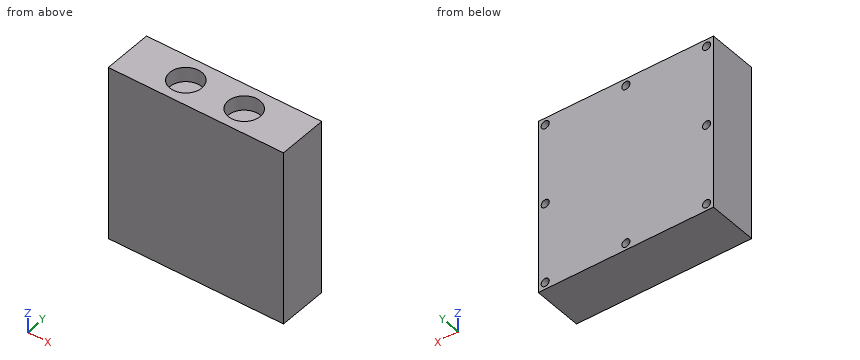
Autodesk Inventor part; units mm, degrees
ref_plane "YZ Plane" through (0, 0, 0) normal (1, 0, 0) x (0, 1, 0)
ref_plane "XZ Plane" through (0, 0, 0) normal (0, 1, 0) x (-1, 0, 0)
ref_plane "XY Plane" through (0, 0, 0) normal (0, 0, 1) x (1, 0, 0)
sketch "Sketch1" plane through (0, 0, 0) normal (0, 1, 0) x (-1, 0, 0)
  line L0 (0, 0) -> (-76.2, 0)
  line L1 (-76.2, 0) -> (-76.2, -76.2)
  line L2 (-76.2, -76.2) -> (0, -76.2)
  line L3 (0, -76.2) -> (0, 0)
  dimension "d0" = 76.2
  dimension "d1" = 76.2
extrude "Extrusion1" add sketch "Sketch1" along normal blind 21.59
sketch "Sketch2" plane through (0, 21.59, 0) normal (0, 1, 0) x (1, 0, 0)
  line L0 (76.2, 76.2) -> (0, 76.2)
  line L1 (38.1, 76.2) -> (38.1, 73.1774)
  line L2 (0, 76.2) -> (0, 0)
  line L3 (0, 38.1) -> (3.0226, 38.1)
  line L4 (0, 0) -> (76.2, 0)
  line L5 (38.1, 0) -> (38.1, 3.0226)
  line L6 (76.2, 0) -> (76.2, 76.2)
  line L7 (76.2, 38.1) -> (73.1774, 38.1)
  circle A0 centre (3.0226, 73.1774) radius 1.7526
  circle A1 centre (73.1774, 3.0226) radius 1.7526
  circle A2 centre (73.1774, 73.1774) radius 1.7526
  circle A3 centre (38.1, 3.0226) radius 1.7526
  circle A4 centre (3.0226, 38.1) radius 1.7526
  circle A5 centre (38.1, 73.1774) radius 1.7526
  circle A6 centre (3.0226, 3.0226) radius 1.7526
  circle A7 centre (73.1774, 38.1) radius 1.7526
  dimension "d5" = 3.0226
  dimension "d6" = 3.0226
  dimension "d7" = 3.0226
  dimension "d8" = 3.0226
  dimension "d9" = 3.5052
  dimension "d10" = 3.5052
  dimension "d11" = 3.5052
  dimension "d12" = 3.5052
  dimension "d13" = 3.5052
  dimension "d14" = 3.5052
  dimension "d15" = 3.5052
  dimension "d16" = 3.5052
extrude "Extrusion2" cut sketch "Sketch2" against normal blind 11.43 contours A5 | A4 | A3 | A7 | A0 | A1 | A2 | A6
sketch "Sketch3" plane through (0, 0, 0) normal (0, 0, 1) x (1, 0, 0)
  line L0 (0, 0) -> (0, 21.59)
  circle A0 centre (25.4, 10.795) radius 6.985
  circle A1 centre (50.8, 10.795) radius 6.985
  dimension "d21" = 13.97
  dimension "d22" = 13.97
extrude "Extrusion3" cut sketch "Sketch3" against normal blind 6.35
properties part number "water_block_top"
Geometry check sheet. Reference: the model listing, model coordinates, mm. Round coordinates to 2 decimals unless told otherwise and drop trailing zeros. Order: outer loops, then holes, each group sorted by start corner. A loop starts at its lowest first (then second) coordinate and runs counter-clockwise, first axis right, second up. Notation, with made-up numbers: (87.5, 39.5) -> (111.5, 39.5) arc R11 cw to (111.5, 55.5) -> close; hole circle Ø2 at (-10.5, 76). An arc over 180 degrees is marked (long way). Return JSON: item names as keys, results as strings. Group by question number.
Q1. Section check B-B, the plane z = -38.1. Record the boundary of the cut face in (x, y), plus the area to 3 significant figures.
Q2. Section check C-C, the plane x = 50.8. Record the boundary of the cut face in (y, z), plus the area to 3 significant figures.
Q3. Gauge pin test, flat ends, axial feed: pin 1 (2 mm diameter, centred on x = 3.02, z = -73.18, fed in from -Y); pin 2 (7 mm diameter, centred on x = 52.5, y = 12.5, fed in from +Z); pin 3 (1.8 mm diameter, centred on x = 2.5, z = -38, fed in from +Y). Record the tip position at first contact, or that the pin passes through.
Q4. Material ranges on probe 1 along X at (y, z) = (18.75, -38.1); probe 2 along Y at (x, z) = (25.4, -1.25); probe 3 along Z at (x, y) = (3.5, 16.25), recorded low to high. Write a range as from..to.
Q5. Section check A-A, the plane x = 38.1. Record the boundary of the cut face in (y, z).
Q6. Section check D-D, the plane x = 23. Record the boundary of the cut face in (y, z).
Numbers:
{
 "1": {"outline": "(0, 0) -> (76.2, 0) -> (76.2, 21.59) -> (74.93, 21.59) -> (74.93, 10.16) -> (71.42, 10.16) -> (71.42, 21.59) -> (4.78, 21.59) -> (4.78, 10.16) -> (1.27, 10.16) -> (1.27, 21.59) -> (0, 21.59) -> close", "area": "1,570 mm^2"},
 "2": {"outline": "(0, -76.2) -> (21.59, -76.2) -> (21.59, 0) -> (17.78, 0) -> (17.78, -6.35) -> (3.81, -6.35) -> (3.81, 0) -> (0, 0) -> close", "area": "1,560 mm^2"},
 "3": {"pin 1": "y = 0", "pin 2": "z = -6.35", "pin 3": "y = 10.16"},
 "4": {"probe 1": "0..1.27, 4.78..71.42, 74.93..76.2", "probe 2": "0..3.81, 17.78..21.59", "probe 3": "-76.2..-74.86, -71.49..-39.79, -36.41..-4.71, -1.34..0"},
 "5": {"outline": "(0, -76.2) -> (21.59, -76.2) -> (21.59, -74.93) -> (10.16, -74.93) -> (10.16, -71.42) -> (21.59, -71.42) -> (21.59, -4.78) -> (10.16, -4.78) -> (10.16, -1.27) -> (21.59, -1.27) -> (21.59, 0) -> (0, 0) -> close"},
 "6": {"outline": "(0, -76.2) -> (21.59, -76.2) -> (21.59, 0) -> (17.35, 0) -> (17.35, -6.35) -> (4.24, -6.35) -> (4.24, 0) -> (0, 0) -> close"}
}
